Read the model definition and answer for the solid it produces. Units are mm, in the model's axes. A direction names the side the tool comes from. Give positions to 0.01 mm unless a question says otherwise; leave off trailing zeros. Loops run counter-clockwise (first coordinate to the right, second up) from the corner with the lowest first, then second, coordinate; pieces in that order, holes last. Notation, with made-up numbers: (34.5, 23.5) -> (83.5, 23.5) arc R17 ccw to (83.5, 42.5) -> close; hole circle Ø5 at (59, -26). An arc over 180 degrees is marked (long way). Return JSON: item names as keys, results as strings. Group by question number.
from build123d import *

# Parameters (mm, degrees)
SKETCH1_W               = 24.51
SKETCH1_H               = 148
BOSS_EXTRUDE1_DEPTH     = 8
SKETCH2_W               = 8
SKETCH2_H               = 148
BOSS_EXTRUDE2_DEPTH     = 25
SKETCH4_W               = 20.3
SKETCH4_H               = 36.8
BOSS_EXTRUDE3_DEPTH     = 8
SKETCH5_W               = 23
SKETCH5_H               = 6
BOSS_EXTRUDE4_DEPTH     = 25
CUT_EXTRUDE2_REACH      = 151.752
SKETCH6_R               = 2
RIB1_REACH              = 159.03
SKETCH8_WALL_W          = 336.456302216
SKETCH8_WALL_H          = 3
MIRROR2_COPY_1_REACH    = 159.03
MIRROR2_COPY_1_SKETCH_W = 336.456302216
MIRROR2_COPY_1_SKETCH_H = 3
SKETCH3_R               = 2.5
CUT_EXTRUDE1_DEPTH      = 10
SKETCH12_R              = 2.75
CUT_EXTRUDE3_DEPTH      = 8
SKETCH13_W              = 5
SKETCH13_H              = 46
BOSS_EXTRUDE5_DEPTH     = 8
SKETCH14_W              = 3
SKETCH14_H              = 17
BOSS_EXTRUDE6_DEPTH     = 8
CHAMFER1_SIZE           = 2
CHAMFER2_SIZE           = 6
CHAMFER2_SIZE2          = 4.047051101
SKETCH15_W              = 33
SKETCH15_H              = 90
CUT_EXTRUDE4_DEPTH      = 48


with BuildPart() as part:
    # Sketch1 → Boss-Extrude1 (new body)
    with BuildSketch(Plane.XY):
        with Locations((-12.255, 74)):
            Rectangle(SKETCH1_W, SKETCH1_H)
    extrude(amount=BOSS_EXTRUDE1_DEPTH)

    # Sketch2 → Boss-Extrude2 (add)
    with BuildSketch(Plane.XY.offset(8)):
        with Locations((-20.51, 74)):
            Rectangle(SKETCH2_W, SKETCH2_H)
    extrude(amount=BOSS_EXTRUDE2_DEPTH)

    # Sketch4 → Boss-Extrude3 (add)
    with BuildSketch(Plane(origin=(0, 0, 0), x_dir=(-1, 0, 0), z_dir=(0, 0, -1))):
        with Locations((-10.15, 129.6)):
            Rectangle(SKETCH4_W, SKETCH4_H)
    extrude(amount=-BOSS_EXTRUDE3_DEPTH)

    # Sketch5 → Boss-Extrude4 (add)
    with BuildSketch(Plane.XY.offset(8)):
        with Locations((8.8, 118.2)):
            Rectangle(SKETCH5_W, SKETCH5_H)
        with Locations((8.8, 141)):
            Rectangle(SKETCH5_W, SKETCH5_H)
    extrude(amount=BOSS_EXTRUDE4_DEPTH)

    # Cut-Extrude2: up to this face of the body (flat: up to its plane)
    cut_extrude2_end = Plane(part.part.faces().sort_by_distance((8.8, 115.2, 20.5))[0])
    # Sketch6 → Cut-Extrude2 (cut, up to the picked face)
    with BuildSketch(Plane(origin=(0, 144, 0), x_dir=(1, 0, 0), z_dir=(0, 1, 0)), mode=Mode.PRIVATE) as cut_extrude2_sk1:
        with Locations(Location((6.6, -20.5, 0), (0, 0, 270))):
            Circle(SKETCH6_R)
    cut_extrude2_tool1 = split(extrude(cut_extrude2_sk1.sketch, amount=-CUT_EXTRUDE2_REACH, mode=Mode.PRIVATE), bisect_by=cut_extrude2_end, keep=Keep.BOTH, mode=Mode.PRIVATE)
    add(cut_extrude2_tool1.solids().sort_by(Axis((6.6, 144, 20.5), (0, -1, 0)))[0], mode=Mode.SUBTRACT)

    # Sketch8 wall → Rib1 (add, up to next)
    with BuildSketch(Plane(origin=(16.3, 146, 18), x_dir=(0, -0.196116135138, 0.980580675691), z_dir=(0, -0.980580675691, -0.196116135138)), mode=Mode.PRIVATE) as rib1_sk1:
        Rectangle(SKETCH8_WALL_W, SKETCH8_WALL_H)
    rib1_tool1 = extrude(rib1_sk1.sketch, amount=RIB1_REACH, mode=Mode.PRIVATE) - part.part
    rib1 = rib1_tool1.solids().sort_by_distance((16.3, 146, 18))[0]
    add(rib1)

    # Mirror1: Rib1 across plane
    add(rib1.mirror(Plane.ZX.offset(129.6)))

    # Mirror2: Rib1 across plane
    add(rib1.mirror(Plane.ZY.offset(-7.55)))

    # Mirror2 copy 1 sketch → Mirror2 copy 1 (add, up to next)
    with BuildSketch(Plane(origin=(-1.2, 113.2, 18), x_dir=(0, 0.196116135138, 0.980580675691), z_dir=(0, 0.980580675691, -0.196116135138)), mode=Mode.PRIVATE) as mirror2_copy_1_sk1:
        Rectangle(MIRROR2_COPY_1_SKETCH_W, MIRROR2_COPY_1_SKETCH_H)
    mirror2_copy_1_tool1 = extrude(mirror2_copy_1_sk1.sketch, amount=MIRROR2_COPY_1_REACH, mode=Mode.PRIVATE) - part.part
    add(mirror2_copy_1_tool1.solids().sort_by_distance((-1.2, 113.2, 18))[0])

    # Sketch3 → Cut-Extrude1 (cut)
    with BuildSketch(Plane.XY.offset(8)):
        with Locations((-8, 8)):
            Circle(SKETCH3_R)
        with Locations((-8, 40)):
            Circle(SKETCH3_R)
        with Locations((-8, 100)):
            Circle(SKETCH3_R)
        with Locations((-8, 132)):
            Circle(SKETCH3_R)
    extrude(amount=-CUT_EXTRUDE1_DEPTH, mode=Mode.SUBTRACT)

    # Sketch12 → Cut-Extrude3 (cut)
    with BuildSketch(Plane.ZY.offset(24.51)):
        with Locations((22, 138.8)):
            Circle(SKETCH12_R)
        with Locations((22, 106.8)):
            Circle(SKETCH12_R)
        with Locations((22, 41.7)):
            Circle(SKETCH12_R)
        with Locations((22, 9.7)):
            Circle(SKETCH12_R)
    extrude(amount=-CUT_EXTRUDE3_DEPTH, mode=Mode.SUBTRACT)

    # Sketch13 → Boss-Extrude5 (add)
    with BuildSketch(Plane(origin=(0, 0, 0), x_dir=(-1, 0, 0), z_dir=(0, 0, -1))):
        with Locations((-2.5, 23)):
            Rectangle(SKETCH13_W, SKETCH13_H)
    extrude(amount=-BOSS_EXTRUDE5_DEPTH)

    # Sketch14 → Boss-Extrude6 (add)
    with BuildSketch(Plane(origin=(0, 0, 0), x_dir=(-1, 0, 0), z_dir=(0, 0, -1))):
        with Locations((-1.5, 102.7)):
            Rectangle(SKETCH14_W, SKETCH14_H)
    extrude(amount=-BOSS_EXTRUDE6_DEPTH)

    # Chamfer1
    chamfer1_edges = [part.edges().sort_by_distance(p)[0] for p in [
        (0, 46, 4),
        (3, 111.2, 4),
        (0, 94.2, 4),
    ]]
    chamfer(chamfer1_edges, length=CHAMFER1_SIZE)

    # Chamfer2
    chamfer2_edges = [part.edges().sort_by_distance(p)[0] for p in [
        (8.8, 121.2, 8),
        (8.8, 138, 8),
    ]]
    chamfer2_side = [part.faces().sort_by_distance(p)[0] for p in [
        (-4.974591741, 76.782250606, 8),
    ]]
    chamfer(chamfer2_edges, length=CHAMFER2_SIZE, length2=CHAMFER2_SIZE2, reference=chamfer2_side[0])

    # Sketch15 → Cut-Extrude4 (cut)
    with BuildSketch(Plane(origin=(20.3, 0, 0), x_dir=(0, 0, -1), z_dir=(1, 0, 0))):
        with Locations((-16.5, 45)):
            Rectangle(SKETCH15_W, SKETCH15_H)
    extrude(amount=-CUT_EXTRUDE4_DEPTH, mode=Mode.SUBTRACT)


solid = part.part
1. Straight lines are drawn through the part: line 1 (Y direction, x = -20, z = 22); line 2 (Y direction, x = -8, z = 4); line 3 (X direction, y = 138.5, z = 15). For each, find the intervals that lie inside material, in ascending order. Write a range as from..to.
2. Which of the six approach directions +Z, -Z, +X, -X, +Y, -Y give full straight-line access (tool end or side, diameter ignored) to faces 4 (the flat face through (19, 113, 8)), 5 (the flat face through (19, 146, 8)), 6 (the flat face through (0, 91, 4)), 7 (the flat face through (8, 146, 8)), 8 (the flat face through (0.3, 114, 15))?
3. Section D-D on y = 100 is taken. Determine the outline of the cut face in (x, z), then the cut area to 3 significant figures.
4. Section B-B on z = 30 is taken. Determine the outline of the cut face in (x, y), then the cut area to 3 significant figures.
5. Flat-ended cylindrical pins translate along their axes: pin 1 Ø6.5 at (x, y) = (-8, 100) entering from -Z; pin 2 Ø1.2 at (y, z) = (112.5, 22.5) entering from +X; pin 3 Ø1 at (y, z) = (112.5, 10.5) entering from +X; pin 4 Ø8 at (x, z) = (15, 10) entering from -Y. Find the tip coordinate at first contact, or state that the pin passes through.
6. Determine the mould class of faces 1 (the flat face through (20.3, 125, 9)), 2 (the flat face through (-16.51, 119, 20)), 3 (the cylindrical face through (-20.566, 105.127, 19.818)) for opening direction X: pulls with the +X half, pulls with the -X half, needs draft (parallel to the pull), parting line crosses it, or undercut.
7. Section C-C on x = -8 is taken. Determine the outline of the cut face in (y, z), then the cut area to 3 significant figures.
8. Section A-A on y = 138.8 is taken. Determine the outline of the cut face in (x, z).
Completed:
{
 "1": {"line 1": "y = 90..104.05, 109.55..136.05, 141.55..148", "line 2": "y = 90..97.5, 102.5..129.5, 134.5..148", "line 3": "x = -24.51..-16.51, -2.7..20.3"},
 "2": {"face 4": "+Z, +X, -Y", "face 5": "+Z, +X, +Y", "face 6": "+Z, -Z, +X, -Y", "face 7": "+Z, +Y", "face 8": "+Z, -Y"},
 "3": {"outline": "(-24.51, 0) -> (-10.5, 0) -> (-10.5, 8) -> (-16.51, 8) -> (-16.51, 33) -> (-24.51, 33) -> close; (-5.5, 0) -> (3, 0) -> (3, 8) -> (-5.5, 8) -> close", "area": "380 mm²"},
 "4": {"outline": "(-24.51, 90) -> (-16.51, 90) -> (-16.51, 148) -> (-24.51, 148) -> close; (-2.7, 115.2) -> (20.3, 115.2) -> (20.3, 121.2) -> (-2.7, 121.2) -> close; (-2.7, 138) -> (20.3, 138) -> (20.3, 144) -> (-2.7, 144) -> close", "area": "740 mm²"},
 "5": {"pin 1": "stops at z = 0", "pin 2": "stops at x = -16.51", "pin 3": "stops at x = 17.8", "pin 4": "stops at y = 111.2"},
 "6": {"face 1": "pulls with the +X half", "face 2": "undercut", "face 3": "needs draft"},
 "7": {"outline": "(90, 0) -> (97.5, 0) -> (97.5, 8) -> (90, 8) -> close; (102.5, 0) -> (129.5, 0) -> (129.5, 8) -> (102.5, 8) -> close; (134.5, 0) -> (148, 0) -> (148, 8) -> (134.5, 8) -> close", "area": "384 mm²"},
 "8": {"outline": "(-24.51, 0) -> (20.3, 0) -> (20.3, 33) -> (-2.7, 33) -> (-2.7, 8) -> (-16.51, 8) -> (-16.51, 19.25) -> (-24.51, 19.25) -> close; (-24.51, 24.75) -> (-16.51, 24.75) -> (-16.51, 33) -> (-24.51, 33) -> close; hole circle Ø4 at (6.6, 20.5)"}
}
